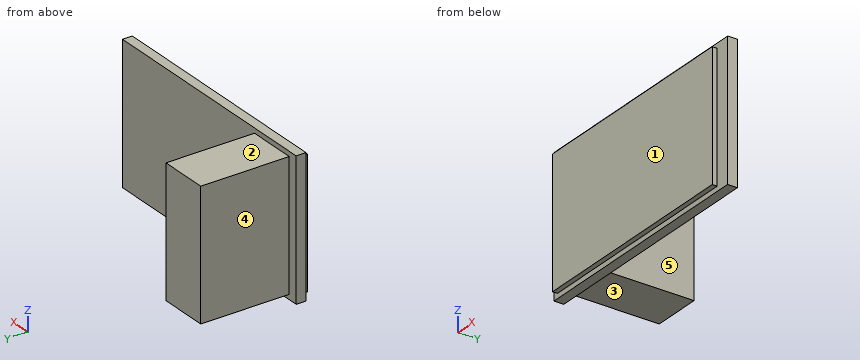
```python
from build123d import *

# Parameters (mm, degrees)
BOX002_W     = 5
BOX002_H     = 10
BOX002_DEPTH = 13
BOX001_W     = 23
BOX001_H     = 1
BOX001_DEPTH = 13
BOX_W        = 25
BOX_H        = 1
BOX_DEPTH    = 14


with BuildPart() as cubo002:
    # Box002 → Box002 (new body)
    with BuildSketch(Plane(origin=(1, 0, 0.5), x_dir=(1, 0, 0), z_dir=(0, 0, 1))):
        with Locations((2.5, 5)):
            Rectangle(BOX002_W, BOX002_H)
    extrude(amount=BOX002_DEPTH)


with BuildPart() as cubo001:
    # Box001 → Box001 (new body)
    with BuildSketch(Plane(origin=(0.5, -0.5, 0.5), x_dir=(1, 0, 0), z_dir=(0, 0, 1))):
        with Locations((11.5, 0.5)):
            Rectangle(BOX001_W, BOX001_H)
    extrude(amount=BOX001_DEPTH)


with BuildPart() as fusion:
    # Box → Box (new body)
    with BuildSketch(Plane.XY):
        with Locations((12.5, 0.5)):
            Rectangle(BOX_W, BOX_H)
    extrude(amount=BOX_DEPTH)

    # Fusion: union Cubo002, Cubo001
    add(cubo002.part)
    add(cubo001.part)


solid = fusion.part
```
Design review of the part built by this model. Coordinates are the model's own, in mm. Face numbers are marked on the shaded views. A direction names the side the tool comes from. Round coordinates to 2 decimals unless told otherwise and drop trailing zeros. Order: outer loops, then holes, each group sorted by start corner. A loop starts at its lowest first (then second) coordinate and runs counter-clockwise, first axis right, second up. Notation, with made-up numbers: (11, 81.25) - (38, 81.25) arc R28 cw to (38, 110.25) - close; hole circle Ø1 at (-15.75, 26). An arc over 180 degrees is marked (long way). One line per question, with ' | ' between items.
Item 1: For P1, Ø2.5, axis at x = 3, y = 6, coming from the -Z side; P2, Ø1.5, axis at x = 16.5, z = 5, coming from the +Y side; P3, Ø2.5, axis at y = 6, z = 8, coming from the +X side, all flat-tipped, find the tip position at first contact; note any pin that passes through.
Checks:
P1: z = 0.5 | P2: y = 1 | P3: x = 6
Item 2: Take a section at C-C, the plane y = 6.5. Write out the cut boundary in (x, z), then the cut area to 3 significant figures.
Checks:
outline: (1, 0.5) - (6, 0.5) - (6, 13.5) - (1, 13.5) - close | area: 65.0 mm²
Item 3: Wall thickness on line 1 (Y direction, x = 22.25, z = 3.5); line 2 (Y direction, x = 24.25, z = 2); line 3 (X direction, y = 8.25, z = 9.25): over which ranges is each line inside the solid? List them lowest first. Write a range as [from, to].
Checks:
line 1: [-0.5, 1] | line 2: [0, 1] | line 3: [1, 6]
Item 4: Machinability: for the marked faces 1, 2, 3, 4 and 5, which of the approach directions +Z, -Z, +X, -X, +Y, -Y give a long, thin tool a straight path to every point of the face, cutting with its end or side? Answer none if there is none.
Checks:
face 1: +Z, -Z, +X, -X, -Y | face 2: +Z, +X, -X, +Y | face 3: -Z, +X, -X, +Y | face 4: +Z, -Z, -X, +Y | face 5: +Z, -Z, +X, +Y
Item 5: Take a section at A-A, the plane x = 7. Write out the cut boundary in (y, z).
Checks:
outline: (-0.5, 0.5) - (0, 0.5) - (0, 0) - (1, 0) - (1, 14) - (0, 14) - (0, 13.5) - (-0.5, 13.5) - close
Item 6: Take a section at B-B, the plane z = 6.5. Write out the cut boundary in (x, y).
Checks:
outline: (0, 0) - (0.5, 0) - (0.5, -0.5) - (23.5, -0.5) - (23.5, 0) - (25, 0) - (25, 1) - (6, 1) - (6, 10) - (1, 10) - (1, 1) - (0, 1) - close
